```python
from build123d import *

# Parameters (mm, degrees)
SKETCH1_R           = 4.7625
BOSS_EXTRUDE1_DEPTH = 102.108
SKETCH2_R           = 3.81
BOSS_EXTRUDE2_DEPTH = 1.016
SKETCH3_R           = 4.7625
BOSS_EXTRUDE3_DEPTH = 5.08
SKETCH4_R           = 3.81
BOSS_EXTRUDE4_DEPTH = 1.016
SKETCH5_R           = 4.7625
BOSS_EXTRUDE5_DEPTH = 5.08


with BuildPart() as part:
    # Sketch1 → Boss-Extrude1 (new body)
    with BuildSketch(Plane.XY):
        Circle(SKETCH1_R)
    extrude(amount=BOSS_EXTRUDE1_DEPTH)

    # Sketch2 → Boss-Extrude2 (add)
    with BuildSketch(Plane(origin=(0, 0, 0), x_dir=(-1, 0, 0), z_dir=(0, 0, -1))):
        Circle(SKETCH2_R)
    extrude(amount=BOSS_EXTRUDE2_DEPTH)

    # Sketch3 → Boss-Extrude3 (add)
    with BuildSketch(Plane(origin=(0, 0, -1.016), x_dir=(-1, 0, 0), z_dir=(0, 0, -1))):
        Circle(SKETCH3_R)
    extrude(amount=BOSS_EXTRUDE3_DEPTH)

    # Sketch4 → Boss-Extrude4 (add)
    with BuildSketch(Plane.XY.offset(102.108)):
        Circle(SKETCH4_R)
    extrude(amount=BOSS_EXTRUDE4_DEPTH)

    # Sketch5 → Boss-Extrude5 (add)
    with BuildSketch(Plane.XY.offset(103.124)):
        Circle(SKETCH5_R)
    extrude(amount=BOSS_EXTRUDE5_DEPTH)


solid = part.part
```
Could you check a few things on this model? Use its own coordinates, in mm. A direction names the side the tool comes from. Round coordinates to 2 decimals unless told otherwise and drop trailing zeros. Loops run counter-clockwise (first coordinate to the right, second up) from the corner with the lowest first, then second, coordinate; pieces in that order, holes last. Notation, with made-up numbers: (55.25, -22.5) - (75.25, -22.5) arc R5 cw to (75.25, -16.5) - close; hole circle Ø8 at (66, -36). An arc over 180 degrees is marked (long way). Answer as CSV lines item,"result".
1. I want a section at B-B on y = 1. List the corners of the cut face in (x, z) for me, then the cut area to 3 significant figures.
Filled in:
outline,"(-4.66, -6.1) - (4.66, -6.1) - (4.66, -1.02) - (3.68, -1.02) - (3.68, 0) - (4.66, 0) - (4.66, 102.11) - (3.68, 102.11) - (3.68, 103.12) - (4.66, 103.12) - (4.66, 108.2) - (-4.66, 108.2) - (-4.66, 103.12) - (-3.68, 103.12) - (-3.68, 102.11) - (-4.66, 102.11) - (-4.66, 0) - (-3.68, 0) - (-3.68, -1.02) - (-4.66, -1.02) - close"
area,"1,060 mm^2"
2. Please list where these lines run through material, in increasing order: line 1 along Z through (x, y) = (-4, 1.5); line 2 along Y through (x, z) = (-0.25, 15.5); line 3 along Y through (x, z) = (3.5, 26). Write a range as [from, to].
Filled in:
line 1,"z = [-6.1, -1.02], [0, 102.11], [103.12, 108.2]"
line 2,"y = [-4.76, 4.76]"
line 3,"y = [-3.23, 3.23]"
3. We'd pull the mould along Z, two halves only. Please class faces 3 (the face through (3.78, -2.9, -3.52)), 4 (the face through (1, 4, 102.108)), 5 (the face through (0, 0, -6.096)): +Z half, -Z half, draft (parallel to the pull), parting line (faces both ways), or undercut.
Filled in:
face 3,"draft"
face 4,"undercut"
face 5,"-Z half"
4. I want a section at A-A on x = 2.5. List the corners of the cut face in (y, z) for me.
Filled in:
outline,"(-4.05, -6.1) - (4.05, -6.1) - (4.05, -1.02) - (2.88, -1.02) - (2.88, 0) - (4.05, 0) - (4.05, 102.11) - (2.88, 102.11) - (2.88, 103.12) - (4.05, 103.12) - (4.05, 108.2) - (-4.05, 108.2) - (-4.05, 103.12) - (-2.88, 103.12) - (-2.88, 102.11) - (-4.05, 102.11) - (-4.05, 0) - (-2.88, 0) - (-2.88, -1.02) - (-4.05, -1.02) - close"
5. I want a section at C-C on z = 47.5. List the corners of the cut face in (x, y) for me (1 decimal).
Filled in:
outline,"circle Ø9.5 at (0, 0)"
6. For pin 1 Ø1.5 at (y, z) = (1, 13) entering from -X; pin 2 Ø1 at (y, z) = (-4, 42.5) entering from +X, each with a flat end and sliding along its axis, tell me the tip position at first contact or that it passes through.
Filled in:
pin 1,"stops at x = -4.76"
pin 2,"stops at x = 3.23"
7. On a 3-axis mill with a long thin cutter (end or side, diameter ignored), from which of +Z, -Z, +X, -X, +Y, -Y can I reach the whole of each face in a straight line? I mean faces 1 (the face through (0, 0, 108.204)), 2 (the face through (1, 4, 103.124)). Say none if no direction works.
Filled in:
face 1,"+Z, +X, -X, +Y, -Y"
face 2,"none"
